from build123d import *

# Parameters (mm, degrees)
EXTRUSION_BASE_SKETCH_W      = 231.5
EXTRUSION_BASE_SKETCH_H      = 40
EXTRUSION_BASE_SKETCH_R      = 2.65
EXTRUSION_BASE_EXTRUDE_DEPTH = 3


with BuildPart() as part:
    # Extrusion Base Sketch → Extrusion Base Extrude (new body)
    with BuildSketch(Plane.XY):
        with Locations((93.75, 16.75)):
            Rectangle(EXTRUSION_BASE_SKETCH_W, EXTRUSION_BASE_SKETCH_H)
        with Locations((-14, 26.75)):
            Circle(EXTRUSION_BASE_SKETCH_R, mode=Mode.SUBTRACT)
        with Locations((-14, 6.75)):
            Circle(EXTRUSION_BASE_SKETCH_R, mode=Mode.SUBTRACT)
        with Locations((201.5, 26.75)):
            Circle(EXTRUSION_BASE_SKETCH_R, mode=Mode.SUBTRACT)
        with Locations((201.5, 6.75)):
            Circle(EXTRUSION_BASE_SKETCH_R, mode=Mode.SUBTRACT)
    extrude(amount=-EXTRUSION_BASE_EXTRUDE_DEPTH)


solid = part.part
Part model, mm, in its own coordinate system. Coordinates: 2 decimals unless noted, no trailing zeros. Write each loop counter-clockwise with the first axis right and the second up, starting at its lowest first coordinate (ties: lowest second). Pieces come first, ordered by that corner, then holes. Notation, with made-up numbers: M 82,15.5 L 113,15.5 A29 ccw 113,53.5 Z; hole C 70,89 d1. An arc over 180 degrees is marked long. Return JSON: item names as keys, results as strings.
1. Saw through at B-B, the plane y = 26.75. Write the cut outline in (x, z).
Determined:
{"outline": "M -22,-3 L -16.65,-3 L -16.65,0 L -22,0 Z; M -11.35,-3 L 198.85,-3 L 198.85,0 L -11.35,0 Z; M 204.15,-3 L 209.5,-3 L 209.5,0 L 204.15,0 Z"}
2. Flat gauge pin, fed straight in: pin 1 Ø5 at (x, y) = (-14, 26.75) entering from -Z. Where does the tip first touch, or does it go through?
Determined:
{"pin 1": "through"}
3. Probe L1, parallel to Y at x = -14, z = -1.6; L2, parallel to X at y = 29, z = -0.5. List the from-to ranges inside material, lowest first.
Determined:
{"L1": "-3.25 to 4.1, 9.4 to 24.1, 29.4 to 36.75", "L2": "-22 to -15.4, -12.6 to 200.1, 202.9 to 209.5"}
4. Pull direction Y, two halves, no side cores. Call faces 1 (the face through (92, 17, -3)), 2 (the face through (-11.55, 5.74, -1.48)): pulls with the +Y half, pulls with the -Y half, needs draft (parallel to the pull), parting line crosses it, or undercut.
Determined:
{"face 1": "needs draft", "face 2": "undercut"}
5. Saw through at A-A, the plane x = -14. Write the cut outline in (y, z).
Determined:
{"outline": "M -3.25,-3 L 4.1,-3 L 4.1,0 L -3.25,0 Z; M 9.4,-3 L 24.1,-3 L 24.1,0 L 9.4,0 Z; M 29.4,-3 L 36.75,-3 L 36.75,0 L 29.4,0 Z"}
